Could you check a few things on this model? Use its own coordinates, in mm. A direction names the side the tool comes from. Round coordinates to 2 decimals unless told otherwise and drop trailing zeros. Write each loop counter-clockwise with the first axis right and the second up, starting at its lowest first coordinate (ties: lowest second). Pieces come first, ordered by that corner, then holes. Notation, with made-up numbers: (81, 40.5) -> (117, 40.5) arc R14 cw to (117, 58.5) -> close; hole circle Ø11 at (39.25, 29). An arc over 180 degrees is marked (long way). Answer in a Markdown table with one row per item. Add a question column.
```python
from build123d import *

# Parameters (mm, degrees)
BOSS_EXTRU_1_DEPTH           = 20
ENL_V_MAT_EXTRU_1_DEPTH      = 334.887542768
ENL_V_MAT_EXTRU_1_DEPTH_BACK = 249
ENL_V_MAT_EXTRU_2_DEPTH      = 334.887542768
ENL_V_MAT_EXTRU_2_DEPTH_BACK = 249
ENL_V_MAT_EXTRU_3_DEPTH      = 315.78213111
ENL_V_MAT_EXTRU_3_DEPTH_BACK = 249
ENL_V_MAT_EXTRU_4_DEPTH      = 315.78213111
ENL_V_MAT_EXTRU_4_DEPTH_BACK = 249
ENL_V_MAT_EXTRU_5_DEPTH      = 334.887542768
ENL_V_MAT_EXTRU_5_DEPTH_BACK = 249
ENL_V_MAT_EXTRU_6_DEPTH      = 334.887542768
ENL_V_MAT_EXTRU_6_DEPTH_BACK = 249
ENL_V_MAT_EXTRU_7_DEPTH      = 315.78213111
ENL_V_MAT_EXTRU_7_DEPTH_BACK = 249
ENL_V_MAT_EXTRU_8_DEPTH      = 315.78213111
ENL_V_MAT_EXTRU_8_DEPTH_BACK = 249


with BuildPart() as part:
    # Esquisse1 → Boss.-Extru.1 (new body)
    with BuildSketch(Plane.XY):
        Polygon((-179.143216373, 44.164624039), (69.856783627, 44.164624039), (69.856783627, 38.864624039), (75.156783627, 38.864624039), (75.156783627, -210.135375961), (69.856783627, -210.135375961), (69.856783627, -215.435375961), (-179.143216373, -215.435375961), (-179.143216373, -210.135375961), (-184.443216373, -210.135375961), (-184.443216373, 38.864624039), (-179.143216373, 38.864624039), align=None)
    extrude(amount=BOSS_EXTRU_1_DEPTH)

    # Esquisse2 → Enlèv. mat.-Extru.1 (cut, two sides: drawn at the far end of the back side and taken through both)
    with BuildSketch(Plane.ZY.offset(179.143216373).offset(-ENL_V_MAT_EXTRU_1_DEPTH_BACK)):
        Polygon((-529.816054004, 38.864624039), (0, 38.864624039), (7.55, 38.864624039), (7.55, 40.414624039), (3.85, 40.414624039), (3.85, 41.414624039), (7.35, 44.164624039), (423.954079466, 371.496400762), (75.014402763, 1372.026913212), (-878.755730707, 1039.395136489), align=None)
    extrude(amount=ENL_V_MAT_EXTRU_1_DEPTH + ENL_V_MAT_EXTRU_1_DEPTH_BACK, mode=Mode.SUBTRACT)

    # Esquisse3 → Enlèv. mat.-Extru.2 (cut, two sides: drawn at the far end of the back side and taken through both)
    with BuildSketch(Plane.ZY.offset(179.143216373).offset(-ENL_V_MAT_EXTRU_2_DEPTH_BACK)):
        Polygon((549.816054004, 38.864624039), (20, 38.864624039), (12.45, 38.864624039), (12.45, 40.414624039), (16.15, 40.414624039), (16.15, 41.414624039), (12.65, 44.164624039), (-403.954079466, 371.496400762), (-55.014402763, 1372.026913212), (898.755730707, 1039.395136489), align=None)
    extrude(amount=ENL_V_MAT_EXTRU_2_DEPTH + ENL_V_MAT_EXTRU_2_DEPTH_BACK, mode=Mode.SUBTRACT)

    # Esquisse5 → Enlèv. mat.-Extru.3 (cut, two sides: drawn at the far end of the back side and taken through both)
    with BuildSketch(Plane(origin=(0, -210.135375961, 0), x_dir=(-1, 0, 0), z_dir=(0, -1, 0)).offset(-ENL_V_MAT_EXTRU_3_DEPTH_BACK)):
        Polygon((179.143216373, 529.816054004), (179.143216373, 0), (179.143216373, -7.55), (180.693216373, -7.55), (180.693216373, -3.85), (181.693216373, -3.85), (184.443216373, -7.35), (511.774993096, -423.954079466), (1512.305505546, -75.014402763), (1179.673728823, 878.755730707), align=None)
    extrude(amount=ENL_V_MAT_EXTRU_3_DEPTH + ENL_V_MAT_EXTRU_3_DEPTH_BACK, mode=Mode.SUBTRACT)

    # Esquisse6 → Enlèv. mat.-Extru.4 (cut, two sides: drawn at the far end of the back side and taken through both)
    with BuildSketch(Plane(origin=(0, -210.135375961, 0), x_dir=(-1, 0, 0), z_dir=(0, -1, 0)).offset(-ENL_V_MAT_EXTRU_4_DEPTH_BACK)):
        Polygon((511.774993096, 403.954079466), (184.443216373, -12.65), (181.693216373, -16.15), (180.693216373, -16.15), (180.693216373, -12.45), (179.143216373, -12.45), (179.143216373, -20), (179.143216373, -549.816054004), (1179.673728823, -898.755730707), (1512.305505546, 55.014402763), align=None)
    extrude(amount=ENL_V_MAT_EXTRU_4_DEPTH + ENL_V_MAT_EXTRU_4_DEPTH_BACK, mode=Mode.SUBTRACT)

    # Esquisse8 → Enlèv. mat.-Extru.5 (cut, two sides: drawn at the far end of the back side and taken through both)
    with BuildSketch(Plane.ZY.offset(179.143216373).offset(-ENL_V_MAT_EXTRU_5_DEPTH_BACK)):
        Polygon((20, -210.135375961), (12.45, -210.135375961), (12.45, -211.685375961), (16.15, -211.685375961), (16.15, -212.685375961), (12.65, -215.435375961), (20, -215.435375961), align=None)
    extrude(amount=ENL_V_MAT_EXTRU_5_DEPTH + ENL_V_MAT_EXTRU_5_DEPTH_BACK, mode=Mode.SUBTRACT)

    # Esquisse9 → Enlèv. mat.-Extru.6 (cut, two sides: drawn at the far end of the back side and taken through both)
    with BuildSketch(Plane.ZY.offset(179.143216373).offset(-ENL_V_MAT_EXTRU_6_DEPTH_BACK)):
        Polygon((423.954079466, -542.767152684), (7.35, -215.435375961), (3.85, -212.685375961), (3.85, -211.685375961), (7.55, -211.685375961), (7.55, -210.135375961), (0, -210.135375961), (-529.816054004, -210.135375961), (-878.755730707, -1210.665888411), (75.014402763, -1543.297665134), align=None)
    extrude(amount=ENL_V_MAT_EXTRU_6_DEPTH + ENL_V_MAT_EXTRU_6_DEPTH_BACK, mode=Mode.SUBTRACT)

    # Esquisse11 → Enlèv. mat.-Extru.7 (cut, two sides: drawn at the far end of the back side and taken through both)
    with BuildSketch(Plane(origin=(0, 38.864624039, 0), x_dir=(1, 0, 0), z_dir=(0, 1, 0)).offset(-ENL_V_MAT_EXTRU_7_DEPTH_BACK)):
        Polygon((69.856783627, 0), (69.856783627, -7.55), (71.406783627, -7.55), (71.406783627, -3.85), (72.406783627, -3.85), (75.156783627, -7.35), (75.156783627, 0), align=None)
    extrude(amount=ENL_V_MAT_EXTRU_7_DEPTH + ENL_V_MAT_EXTRU_7_DEPTH_BACK, mode=Mode.SUBTRACT)

    # Esquisse12 → Enlèv. mat.-Extru.8 (cut, two sides: drawn at the far end of the back side and taken through both)
    with BuildSketch(Plane(origin=(0, 38.864624039, 0), x_dir=(1, 0, 0), z_dir=(0, 1, 0)).offset(-ENL_V_MAT_EXTRU_8_DEPTH_BACK)):
        Polygon((402.48856035, 403.954079466), (75.156783627, -12.65), (72.406783627, -16.15), (71.406783627, -16.15), (71.406783627, -12.45), (69.856783627, -12.45), (69.856783627, -20), (69.856783627, -549.816054004), (1070.387296077, -898.755730707), (1403.0190728, 55.014402763), align=None)
    extrude(amount=ENL_V_MAT_EXTRU_8_DEPTH + ENL_V_MAT_EXTRU_8_DEPTH_BACK, mode=Mode.SUBTRACT)


solid = part.part
```
(1) Suppose I cut it at B-B, the plane y = -125.5. Please give me the cut outline in (x, z), then the cut area to 3 significant figures.
(2) I need wall thicknesses on L1, parallel to X at y = -40.5, z = 7.5; L2, parallel to Y at x = -95, z = 15.25; L3, parallel to X at y = -145.5, z = 14.5. Which ranges of each line are inside material? Lowest first, please.
(3) If we mould it in two halves opening along Y, with no side actions, what happens to faces 4 (the face through (-179.143, -84, 16)), 5 (the face through (-56, 38.865, 16)), 6 (the face through (-53, -210.135, 16))? For each: pulls with the +Y half, pulls with the -Y half, needs draft (parallel to the pull), parting line crosses it, or undercut.
(4) Suppose I cut it at A-A, the plane x = 46. Please give me the cut outline in (y, z).
(5) For P1, Ø1, axis at y = 8.5, z = 14, coming from the -X side; P2, Ø1.8, axis at y = -68.5, z = 5.5, coming from the -X side; P3, Ø0.5, axis at x = -180, y = -47.5, coming from the -Z side, each with a flat end and sliding along its axis, tell me the tip position at first contact or that it passes through.
(6) On a 3-axis mill with a long thin cutter (end or side, diameter ignored), from which of +Z, -Z, +X, -X, +Y, -Y can I reach the whole of each face in a straight line? I mean faces 1 (the face through (69.857, -87, 16)), 2 (the face through (-56, 38.865, 4)), 3 (the face through (69.857, -87, 4)). Say none if no direction works.
Response:
| question | item | result |
|---|---|---|
| 1 | outline | (-184.44, 7.35) -> (-181.69, 3.85) -> (-180.69, 3.85) -> (-180.69, 7.55) -> (-179.14, 7.55) -> (-179.14, 0) -> (69.86, 0) -> (69.86, 7.55) -> (71.41, 7.55) -> (71.41, 3.85) -> (72.41, 3.85) -> (75.16, 7.35) -> (75.16, 12.65) -> (72.41, 16.15) -> (71.41, 16.15) -> (71.41, 12.45) -> (69.86, 12.45) -> (69.86, 20) -> (-179.14, 20) -> (-179.14, 12.45) -> (-180.69, 12.45) -> (-180.69, 16.15) -> (-181.69, 16.15) -> (-184.44, 12.65) -> close |
| 1 | area | 5,070 mm² |
| 2 | L1 | -184.44 to -180.69, -179.14 to 69.86, 71.41 to 75.16 |
| 2 | L2 | -213.39 to -211.69, -210.14 to 38.86, 40.41 to 42.12 |
| 2 | L3 | -182.99 to -180.69, -179.14 to 69.86, 71.41 to 73.7 |
| 3 | face 4 | needs draft |
| 3 | face 5 | undercut |
| 3 | face 6 | undercut |
| 4 | outline | (-215.44, 7.35) -> (-212.69, 3.85) -> (-211.69, 3.85) -> (-211.69, 7.55) -> (-210.14, 7.55) -> (-210.14, 0) -> (38.86, 0) -> (38.86, 7.55) -> (40.41, 7.55) -> (40.41, 3.85) -> (41.41, 3.85) -> (44.16, 7.35) -> (44.16, 12.65) -> (41.41, 16.15) -> (40.41, 16.15) -> (40.41, 12.45) -> (38.86, 12.45) -> (38.86, 20) -> (-210.14, 20) -> (-210.14, 12.45) -> (-211.69, 12.45) -> (-211.69, 16.15) -> (-212.69, 16.15) -> (-215.44, 12.65) -> close |
| 5 | P1 | x = -183.78 |
| 5 | P2 | x = -183.7 |
| 5 | P3 | z = 7.55 |
| 6 | face 1 | +Z, +Y, -Y |
| 6 | face 2 | -Z, +X, -X |
| 6 | face 3 | -Z, +Y, -Y |
